```python
from build123d import *

# Parameters (mm, degrees)
F1_DEPTH = 50.8
F4_R     = 29.21
F5_DEPTH = 250.19
F6_W     = 161.29
F6_H     = 41.656
F6_H_2   = 62.738
F7_DEPTH = 243.5455460034
F8_D     = 38.1


with BuildPart() as f1:
    # F0 (on Top) → F1 (new body)
    with BuildSketch(Plane.XY):
        with BuildLine():
            ThreePointArc((0, 38.1), (11.1592316368, 11.1592316368), (38.1, 0))
            Line((38.1, 0), (215.9, 0))
            ThreePointArc((215.9, 0), (242.8407683632, 11.1592316368), (254, 38.1))
            Line((254, 38.1), (254, 266.7))
            ThreePointArc((254, 266.7), (242.8407683632, 293.6407683632), (215.9, 304.8))
            Line((215.9, 304.8), (38.1, 304.8))
            ThreePointArc((38.1, 304.8), (11.1592316368, 293.6407683632), (0, 266.7))
            Line((0, 266.7), (0, 38.1))
        make_face()
    extrude(amount=F1_DEPTH)

    # F4 (on line) → F5 (join, through all)
    with BuildSketch(Plane(origin=(77.216, -77.216, 0), x_dir=(-0.7071067812, -0.7071067812, 0), z_dir=(-0.7071067812, 0.7071067812, 0))):
        with BuildLine():
            Line((-234.8987233236, 125.222), (-234.8987233236, 50.8))
            Line((-234.8987233236, 50.8), (-151.5867233236, 50.8))
            Line((-151.5867233236, 50.8), (-151.5867233236, 125.222))
            ThreePointArc((-151.5867233236, 125.222), (-193.2427233236, 166.878), (-234.8987233236, 125.222))
        make_face()
        with Locations((-193.2427233236, 125.222)):
            Circle(F4_R, mode=Mode.SUBTRACT)
    extrude(amount=F5_DEPTH)

    # F6 (on face) → F7 (cut, through all)
    with BuildSketch(Plane(origin=(107.188, 107.188, 0), x_dir=(0.7071067812, -0.7071067812, 0), z_dir=(-0.7071067812, -0.7071067812, 0))):
        with Locations((-15.8950855678, 146.05)):
            Rectangle(F6_W, F6_H)
        with Locations((-15.8950855678, 93.853)):
            Rectangle(F6_W, F6_H_2)
    extrude(amount=-F7_DEPTH, mode=Mode.SUBTRACT)

    # F8 (through all)
    with Locations(Plane.XY.offset(50.8)):
        with Locations((38.1, 38.1), (215.9, 266.7)):
            Hole(F8_D / 2)


solid = f1.part
```
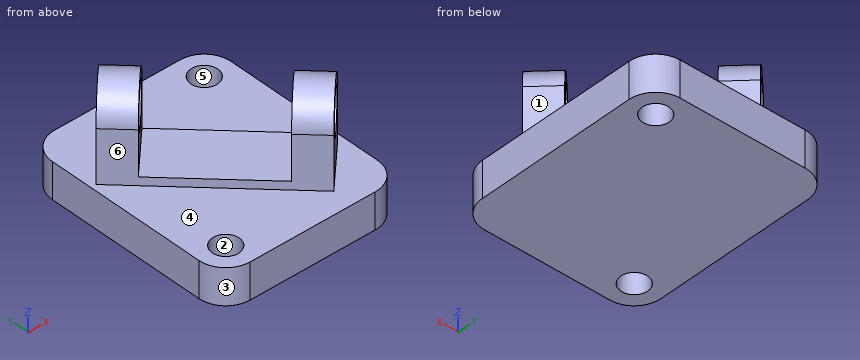
Part model, mm, in its own coordinate system. Face numbers are marked on the shaded views. A direction names the side the tool comes from. Round coordinates to 2 decimals unless told otherwise and drop trailing zeros. Order: outer loops, then holes, each group sorted by start corner. A loop starts at its lowest first (then second) coordinate and runs counter-clockwise, first axis right, second up. Notation, with made-up numbers: M -21,-1.75 L 27,-1.75 A14 ccw 27,11.25 Z; hole C 17,-18 d7. An arc over 180 degrees is marked long. Answer in a Markdown table with one row per item. Add a question column.
Q1. Wall check: L1, parallel to Y at x = 215.9, z = 12; L2, parallel to X at y = 266, z = 27; L3, parallel to Y at x = 38.1, z = 23.5. Give the ranges that are in metal, low to high. Write a range as from..to.
Q2. 3-axis set-ups, long thin cutter, end or side, ignore diameter. For the marked faces 4, 5 and 6: which of +Z, -Z, +X, -X, +Y, -Y reach the whole face in a straight line?
Q3. Cut at B-B on z = 114. Give the cut face in (x, y).
Q4. Cut at C-C on y = 128.5. Give the cut face in (x, z).
Q5. Cut at A-A on z = 74.5. Give the cut face in (x, y), and give its area (3 significant figures).
Q6. Mould opens along X. For the marked faces 1, 2 and 3 say: +X half, -X half, draft (parallel to the pull), parting line (faces both ways), or undercut.
Q7. Pin check, flat tips, straight feed: pin 1 (5 mm diameter, centred on y = 157.5, z = 26.5, fed in from -X); pin 2 (2 mm diameter, centred on x = 205, y = 154.5, fed in from +Z); pin 3 (6 mm diameter, centred on x = 178, z = 56.5, fed in from +Y); pin 4 (23 mm diameter, centred on x = 215.9, y = 266.7, fed in from -Z). Stop position of each tip, or through.
Established:
| question | item | result |
|---|---|---|
| 1 | L1 | y = 0..247.65, 285.75..304.8 |
| 1 | L2 | x = 0..196.86, 234.94..254 |
| 1 | L3 | y = 0..19.05, 57.15..304.8 |
| 2 | face 4 | +Z |
| 2 | face 5 | +Z, -Z |
| 2 | face 6 | +Z, -X, -Y |
| 3 | outline | M 7.49,206.88 L 38.92,175.45 L 49.31,185.84 L 17.88,217.27 Z; M 56.02,255.41 L 87.45,223.98 L 97.83,234.36 L 66.4,265.79 Z; M 152.97,61.4 L 184.4,29.97 L 194.79,40.36 L 163.36,71.79 Z; M 201.5,109.93 L 232.93,78.5 L 243.31,88.88 L 211.88,120.31 Z |
| 4 | outline | M 0,0 L 254,0 L 254,50.8 L 203.7,50.8 L 203.7,62.48 L 85.88,62.48 L 85.88,50.8 L 0,50.8 Z |
| 5 | outline | M 7.49,206.88 L 38.92,175.45 L 97.83,234.36 L 66.4,265.79 Z; M 152.97,61.4 L 184.4,29.97 L 243.31,88.88 L 211.88,120.31 Z |
| 5 | area | 7,410 mm2 |
| 6 | face 1 | +X half |
| 6 | face 2 | undercut |
| 6 | face 3 | -X half |
| 7 | pin 1 | stops at x = 0 |
| 7 | pin 2 | stops at z = 50.8 |
| 7 | pin 3 | stops at y = 157.2 |
| 7 | pin 4 | passes through |
